Work out the finished part from the listing and answer in its coordinate system (mm). A direction names the side the tool comes from. Round coordinates to 2 decimals unless told otherwise and drop trailing zeros. Loops run counter-clockwise (first coordinate to the right, second up) from the corner with the lowest first, then second, coordinate; pieces in that order, holes last. Notation, with made-up numbers: (65, -25) - (80, -25) arc R17 ccw to (80, -9) - close; hole circle Ø7 at (-31, -38). An arc over 180 degrees is marked (long way). Use CSV: the item, a comma, the result in double quotes. Start each with the question number.
from build123d import *

# Parameters (mm, degrees)
BOSS_EXTRUDE1_DEPTH = 16
SKETCH2_R           = 4
CUT_EXTRUDE1_DEPTH  = 19.8
SKETCH3_R           = 1.5
CUT_EXTRUDE2_DEPTH  = 26


with BuildPart() as part:
    # Sketch1 → Boss-Extrude1 (new body)
    with BuildSketch(Plane(origin=(0, 0, 0), x_dir=(1, 0, 0), z_dir=(0, 1, 0))):
        Polygon((-9.4, 0), (9.4, 0), (9.4, -25), (5, -25), (5, -5), (-5, -5), (-5, -25), (-9.4, -25), align=None)
    extrude(amount=BOSS_EXTRUDE1_DEPTH)

    # Sketch2 → Cut-Extrude1 (cut, through all)
    with BuildSketch(Plane(origin=(9.4, 0, 0), x_dir=(0, 0, -1), z_dir=(1, 0, 0))):
        with Locations((-19, 7)):
            Circle(SKETCH2_R)
    extrude(amount=-CUT_EXTRUDE1_DEPTH, mode=Mode.SUBTRACT)

    # Sketch3 → Cut-Extrude2 (cut, through all)
    with BuildSketch(Plane(origin=(0, 0, 0), x_dir=(-1, 0, 0), z_dir=(0, 0, -1))):
        with Locations((0, 13)):
            Circle(SKETCH3_R)
        with Locations((0, 3)):
            Circle(SKETCH3_R)
    extrude(amount=-CUT_EXTRUDE2_DEPTH, mode=Mode.SUBTRACT)


solid = part.part
Item 1: The mould has two halves that part along Y. Classify faces 3 (the flat face through (0, 16, 4)), 4 (the flat face through (0, 8, 5)), 5 (the cylindrical face through (7.2, 4.6, 22.2)): pulls with the +Y half, pulls with the -Y half, needs draft (parallel to the pull), parting line crosses it, or undercut.
Item 2: Which of the six approach directions +Z, -Z, +X, -X, +Y, -Y give full straight-line access (tool end or side, diameter ignored) to faces 1 (the flat face through (-5, 7.9, 14.9)), 2 (the cylindrical face through (0.325, 1.536, 2.465))?
Item 3: Each of these flat-tipped pins is pushed along its axis until it touches: pin 1 Ø3 at (x, z) = (-2.5, 22) entering from -Y; pin 2 Ø8 at (x, y) = (0, 11) entering from +Z. Where does it stop, or does it pass through?
Item 4: A cutting plane is placed at D-D (x = 0). Determine the outline of the cut face in (y, z), plus the area to 3 significant figures.
Item 5: A cutting plane is placed at B-B (z = 19). Determine the outline of the cut face in (x, y).
Item 6: A cutting plane is placed at C-C (y = 13). Determine the outline of the cut face in (x, z).
Item 7: Find the intervals of material crossed by probe 1 along Y at (x, z) = (0, 3.7); probe 2 along X at (y, z) = (14.5, 15.5); probe 3 along Y at (x, z) = (-8.15, 19), in increasing order. Write a range as [from, to].
Item 8: A cutting plane is placed at A-A (y = 7). Determine the outline of the cut face in (x, z).
Result sheet:
1,face 3,"pulls with the +Y half"
1,face 4,"needs draft"
1,face 5,"undercut"
2,face 1,"+Z, +Y, -Y"
2,face 2,"+Z, -Z"
3,pin 1,"through"
3,pin 2,"z = 5"
4,outline,"(0, 0) - (1.5, 0) - (1.5, 5) - (0, 5) - close; (4.5, 0) - (11.5, 0) - (11.5, 5) - (4.5, 5) - close; (14.5, 0) - (16, 0) - (16, 5) - (14.5, 5) - close"
4,area,"50.0 mm^2"
5,outline,"(-9.4, 0) - (-5, 0) - (-5, 3) - (-9.4, 3) - close; (-9.4, 11) - (-5, 11) - (-5, 16) - (-9.4, 16) - close; (5, 0) - (9.4, 0) - (9.4, 3) - (5, 3) - close; (5, 11) - (9.4, 11) - (9.4, 16) - (5, 16) - close"
6,outline,"(-9.4, 0) - (-1.5, 0) - (-1.5, 5) - (-5, 5) - (-5, 25) - (-9.4, 25) - close; (1.5, 0) - (9.4, 0) - (9.4, 25) - (5, 25) - (5, 5) - (1.5, 5) - close"
7,probe 1,"[0, 1.5], [4.5, 11.5], [14.5, 16]"
7,probe 2,"[-9.4, -5], [5, 9.4]"
7,probe 3,"[0, 3], [11, 16]"
8,outline,"(-9.4, 0) - (9.4, 0) - (9.4, 15) - (5, 15) - (5, 5) - (-5, 5) - (-5, 15) - (-9.4, 15) - close; (-9.4, 23) - (-5, 23) - (-5, 25) - (-9.4, 25) - close; (5, 23) - (9.4, 23) - (9.4, 25) - (5, 25) - close"
